Autodesk Inventor part; units mm, degrees
ref_plane "Work Plane1" through (-18, 40, 0) normal (-1, 0, 0) x (0, -1, 0)
ref_plane "YZ Plane" through (0, 0, 0) normal (1, 0, 0) x (0, 1, 0)
ref_plane "XZ Plane" through (0, 0, 0) normal (0, 1, 0) x (-1, 0, 0)
sketch "Sketch1" plane through (0, 0, 0) normal (0, 1, 0) x (-1, 0, 0)
  circle A0 centre (0, 0) radius 16.5
  circle A1 centre (0, 0) radius 18
  dimension "d0" = 33
  dimension "d1" = 36
extrude "Extrusion1" add sketch "Sketch1" along normal blind 40
sketch "Sketch2" plane through (0, 40, 0) normal (0, 1, 0) x (1, 0, 0)
  circle A0 centre (0, 0) radius 18 construction
  circle A1 centre (0, 0) radius 16.5 construction
  line L0 (0, 0) -> (-18, 0) construction
ref_plane "Work Plane1" through (-18, 40, 0) normal (-1, 0, 0) x (0, -1, 0)
sketch "Sketch3" plane through (-18, 40, 0) normal (-1, 0, 0) x (0, -1, 0)
  line L0 (0, 18) -> (0, -18) construction
  line L1 (40, 18) -> (40, -18) construction
  line L2 (0, 0) -> (40, 0)
  line L3 (40, 0) -> (40, -8)
  line L4 (40, -8) -> (0, -8)
  line L5 (0, -8) -> (0, 0)
  line L6 (40, 0) -> (40, 8)
  line L7 (40, 8) -> (0, 8)
  line L8 (0, 8) -> (0, 0)
  line L9 (0, -8) -> (40, -8)
  line L10 (40, -8) -> (40, -14)
  line L11 (40, -14) -> (0, -14)
  line L12 (0, -14) -> (0, -8)
  line L13 (0, 8) -> (40, 8)
  line L14 (40, 8) -> (40, 14)
  line L15 (40, 14) -> (0, 14)
  line L16 (0, 14) -> (0, 8)
  dimension "d4" = 8
  dimension "d5" = 6
  dimension "d6" = 6
extrude "Extrusion2" add sketch "Sketch3" against normal up to surface contours L8 L7 L6 L2 | L2 L3 L4 L5
extrude "Extrusion3" add sketch "Sketch3" along normal blind 1
sketch "Sketch4" plane through (-19, 40, 0) normal (-1, 0, 0) x (0, 0, 1)
  line L0 (14, 0) -> (-14, 0) construction
  line L1 (-14, -40) -> (-10, -40)
  line L2 (-10, -40) -> (-10, 0)
  line L3 (-10, 0) -> (-14, 0)
  line L4 (-14, 0) -> (-14, -40)
  line L5 (-10, 0) -> (10.2529, 0)
  line L6 (10.2529, 0) -> (10.2529, -4)
  line L7 (10.2529, -4) -> (-10, -4)
  line L8 (-10, -4) -> (-10, 0)
  line L9 (14, -40) -> (10, -40)
  line L10 (10, -40) -> (10, 0)
  line L11 (10, 0) -> (14, 0)
  line L12 (14, 0) -> (14, -40)
  line L13 (10, -40) -> (-10, -40)
  line L14 (-10, -40) -> (-10, -36)
  line L15 (-10, -36) -> (10, -36)
  line L16 (10, -36) -> (10, -40)
  point P0 (0, -40)
  point P1 (10, -4)
  point P2 (-10, -4)
  dimension "d11" = 4
  dimension "d12" = 4
  dimension "d13" = 4
  dimension "d14" = 4
extrude "Extrusion4" add sketch "Sketch4" along normal blind 1 contours L4 L3 L2 L1 | L2 L15 L10 L13 | L10 L7 L6 L11 L12 L9 | L5 L10 L7 L2 | L5 L6 L7 L10
Check sheet for the modelled part. Datum: model origin and axes. Units: mm. A direction names the side the tool comes from. Round coordinates to 2 decimals unless told otherwise and drop trailing zeros. Loops run counter-clockwise (first coordinate to the right, second up) from the corner with the lowest first, then second, coordinate; pieces in that order, holes last.
1. Scan lines: probe 1 along Z at (x, y) = (0, 28); probe 2 along X at (y, z) = (29.5, -0.5); probe 3 along X at (y, z) = (5, -13). Record each from-to range of solid material in increasing order.
2. Sectioned sample at A-A on y = 9.5. Record the boundary of the cut face in (x, z).
3. Gauge pin test, flat ends, axial feed: pin 1 Ø3 at (x, z) = (-6.5, 12.5) entering from -Y; pin 2 Ø5 at (x, y) = (-12.5, 33) entering from -Z; pin 3 Ø1.6 at (x, y) = (-19, 17) entering from +Z; pin 4 Ø10 at (y, z) = (22.5, 2) entering from -X. Record the tip position at first contact, or that the pin passes through.
4. Sectioned sample at C-C on z = 0. Record the boundary of the cut face in (x, y).
5. Set-up check for faces 1 (the flat face through (-19, 20, 14)), 2 (the flat face through (-19.5, 19.8, 10)), 3 (the flat face through (-17, 20, -8)), 4 (the flat face through (-18, 20, 11)), 5 (the flat face through (-19, 20, -14)): record each of +Z, -Z, +X, -X, +Y, -Y from which the full face is reachable in a straight line by a thin tool's end or side.
6. Sectioned sample at B-B on x = 0. Record the boundary of the cut face in (y, z), and give its area (3 significant figures).
7. Sectioned sample at D-D on z = 12. Record the boundary of the cut face in (x, y), and give its area (3 significant figures).
8. Mould release check, pull along Y, two halves, no side actions. Record for faces 6 (the flat face through (-19.5, 19.8, -10)), 7 (the cylindrical face through (17.987, 19.72, -0.675)), 8 (the flat face through (-16.4, 0, 3.9)), 9 (the flat face through (-16.4, 40, -3.9)): released by +Y, released by -Y, zero draft, split by the parting line, or undercut.
Recorded:
1. probe 1: z = -18 to -16.5, 16.5 to 18
1. probe 2: x = -19 to -16.49, 16.49 to 17.99
1. probe 3: x = -20 to -18, -12.45 to -10.16, 10.16 to 12.45
2. outline: (-20, -14) - (-18, -14) - (-18, -8) - (-16.12, -8) arc R18 ccw (long way) to (-16.12, 8) - (-18, 8) - (-18, 14) - (-20, 14) - (-20, 10) - (-19, 10) - (-19, -10) - (-20, -10) - close; hole circle Ø33 at (0, 0)
3. pin 1: passes through
3. pin 2: stops at z = -14.97
3. pin 3: stops at z = 14
3. pin 4: stops at x = -19
4. outline: (-20, 0) - (-16.5, 0) - (-16.5, 40) - (-20, 40) - (-20, 36) - (-19, 36) - (-19, 4) - (-20, 4) - close; (16.5, 0) - (18, 0) - (18, 40) - (16.5, 40) - close
5. face 1: +Z, -X, +Y, -Y
5. face 2: -X
5. face 3: -Z, +Y, -Y
5. face 4: +Z, +Y, -Y
5. face 5: -Z, -X, +Y, -Y
6. outline: (0, -18) - (40, -18) - (40, -16.5) - (0, -16.5) - close; (0, 16.5) - (40, 16.5) - (40, 18) - (0, 18) - close
6. area: 120 mm2
7. outline: (-20, 0) - (-18, 0) - (-18, 40) - (-20, 40) - close; (-13.42, 0) - (-11.32, 0) - (-11.32, 40) - (-13.42, 40) - close; (11.32, 0) - (13.42, 0) - (13.42, 40) - (11.32, 40) - close
7. area: 247 mm2
8. face 6: undercut
8. face 7: zero draft
8. face 8: released by -Y
8. face 9: released by +Y
